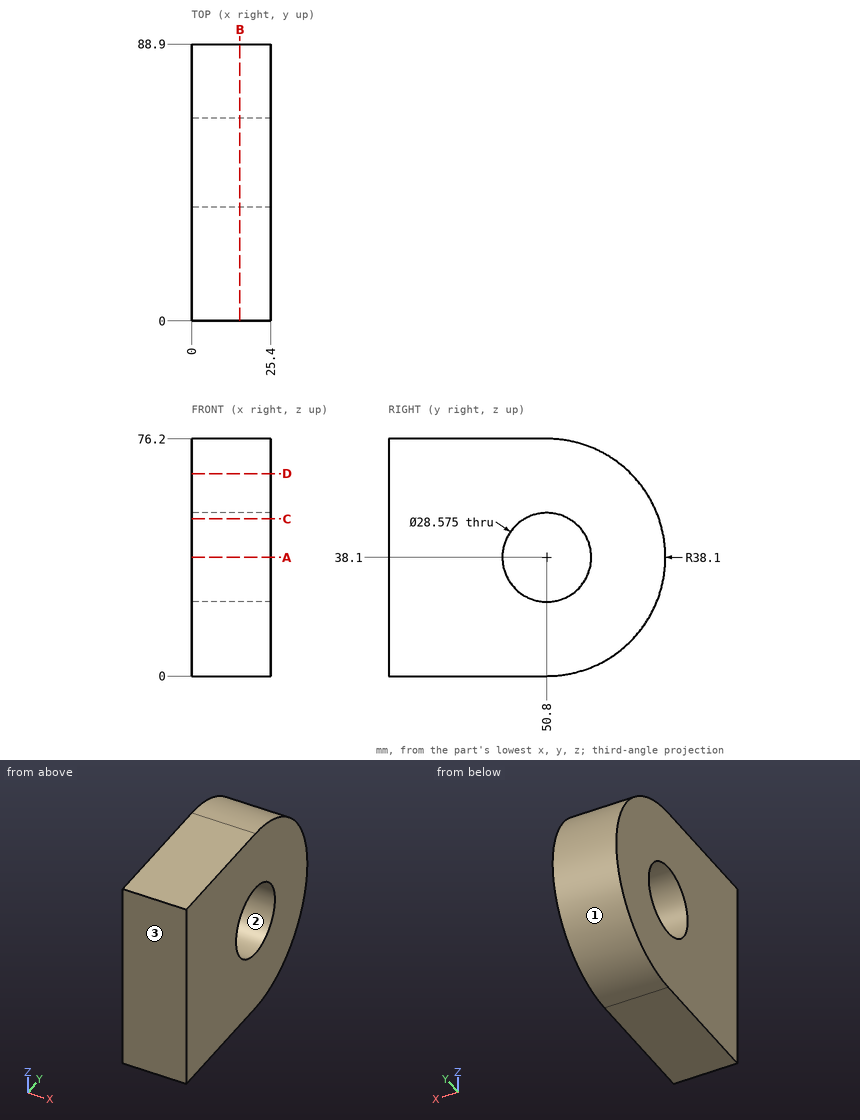
The drawing under review shows one solid part. Ordinate dimensions are in mm from its lowest x, y, z. Round coordinates to 2 decimals unless told otherwise and drop trailing zeros. Write each loop counter-clockwise with the first axis right and the second up, starting at its lowest first coordinate (ties: lowest second). Pieces come first, ordered by that corner, then holes. Notation, with made-up numbers: M -30,-17.5 L -13,-17.5 A15 ccw -13,-5.5 Z; hole C 7,-15.5 d9. An arc over 180 degrees is marked long. One line per item, written item: value. Start each with the question number.
(1) The part is to be moulded in two halves that separate along Z. For the marked faces 1, 2 and 3, say which applies: released by +Z, released by -Z, zero draft, split by the parting line, or undercut.
(2) Wall thickness on line 1 (Y direction, x = 5.5, z = 38.1); line 2 (Z direction, x = 16.5, y = 54); line 3 (Z direction, x = 8.25, y = 54.5): over which ranges is each line inside the solid? List them lowest first.
(3) We need section B-B (x = 15.5). Give the boundary of the cut face in (y, z) (1 decimal).
(4) We need section D-D (z = 65). Give the boundary of the cut face in (x, y).
(5) Insertion check: pin 1 (8 mm diameter, centred on x = 10, z = 23.5, fed in from +Y). The pin has a flat end and moves straight along its axis. Give the tip position at first contact, or say it passes through.
(6) We need section A-A (z = 38.1). Give the boundary of the cut face in (x, y).
(7) We need section C-C (z = 50.5). Give the boundary of the cut face in (x, y).
Result:
1. face 1: split by the parting line
1. face 2: undercut
1. face 3: zero draft
2. line 1: 0 to 36.51, 65.09 to 88.9
2. line 2: 0.13 to 24.18, 52.02 to 76.07
2. line 3: 0.18 to 24.3, 51.9 to 76.02
3. outline: M 0,0 L 50.8,0 A38.1 ccw 50.8,76.2 L 0,76.2 Z; hole C 50.8,38.1 d28.6
4. outline: M 0,0 L 25.4,0 L 25.4,77.78 L 0,77.78 Z
5. pin 1: y = 87.4
6. outline: M 0,0 L 25.4,0 L 25.4,36.51 L 0,36.51 Z; M 0,65.09 L 25.4,65.09 L 25.4,88.9 L 0,88.9 Z
7. outline: M 0,0 L 25.4,0 L 25.4,43.7 L 0,43.7 Z; M 0,57.9 L 25.4,57.9 L 25.4,86.83 L 0,86.83 Z
